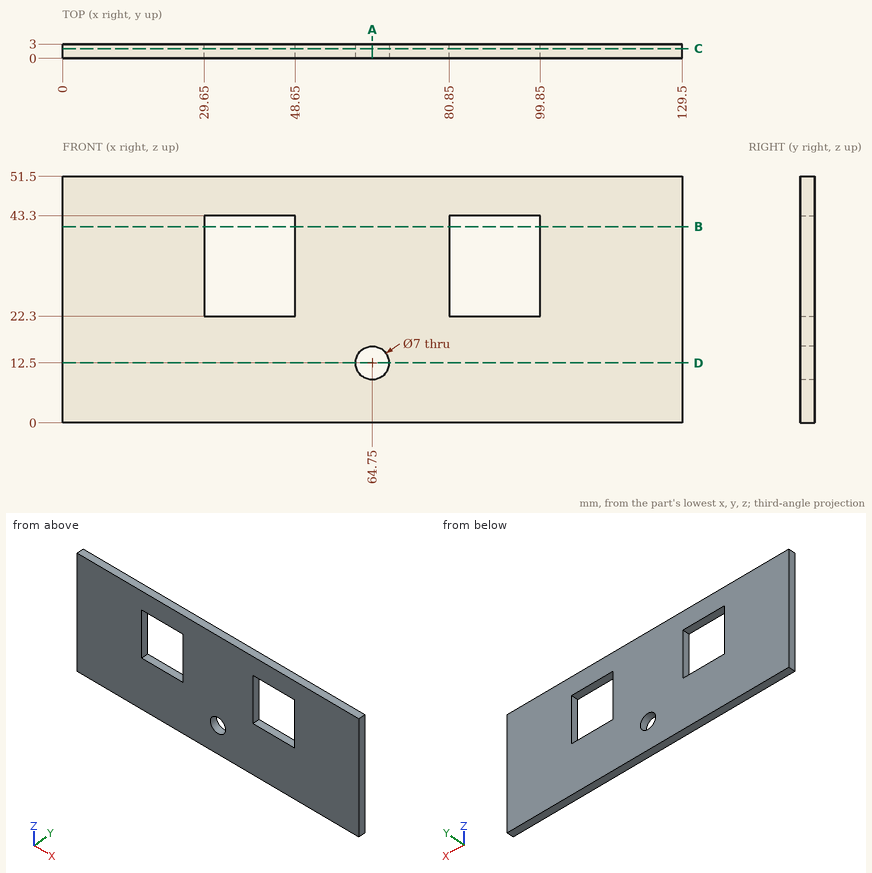
Print and shaded views of the part. All mm, measured from the part's lowest x, y and z. Coordinates: 2 decimals unless noted, no trailing zeros. Order: outer loops, then holes, each group sorted by start corner. A loop starts at its lowest first (then second) coordinate and runs counter-clockwise, first axis right, second up.
(1) Slice it at A-A, the plane x = 64.75. Write the cut outline in (y, z), and give its area (4 significant figures).
Check sheet entries:
outline: (0, 0) - (3, 0) - (3, 9) - (0, 9) - close; (0, 16) - (3, 16) - (3, 51.5) - (0, 51.5) - close
area: 133.5 mm2
(2) Slice it at D-D, the plane z = 12.5. Write the cut outline in (x, y), and give its area (4 significant figures).
Check sheet entries:
outline: (0, 0) - (61.25, 0) - (61.25, 3) - (0, 3) - close; (68.25, 0) - (129.5, 0) - (129.5, 3) - (68.25, 3) - close
area: 367.5 mm2
(3) Probe L1, parallel to X at y = 1.55, z = 41; L2, parallel to Z at x = 64.75, y = 1.45; L3, parallel to Z at x = 42, y = 1.1. List the from-to ranges inside material, lowest first.
Check sheet entries:
L1: x = 0 to 29.65, 48.65 to 80.85, 99.85 to 129.5
L2: z = 0 to 9, 16 to 51.5
L3: z = 0 to 22.3, 43.3 to 51.5
(4) Slice it at C-C, the plane y = 2.05. Write the cut outline in (x, z), and give its area (3 significant figures).
Check sheet entries:
outline: (0, 0) - (129.5, 0) - (129.5, 51.5) - (0, 51.5) - close; hole (29.65, 22.3) - (48.65, 22.3) - (48.65, 43.3) - (29.65, 43.3) - close; hole circle Ø7 at (64.75, 12.5); hole (80.85, 22.3) - (99.85, 22.3) - (99.85, 43.3) - (80.85, 43.3) - close
area: 5,830 mm2
(5) Slice it at B-B, the plane z = 41. Write the cut outline in (x, y), and give its area (4 significant figures).
Check sheet entries:
outline: (0, 0) - (29.65, 0) - (29.65, 3) - (0, 3) - close; (48.65, 0) - (80.85, 0) - (80.85, 3) - (48.65, 3) - close; (99.85, 0) - (129.5, 0) - (129.5, 3) - (99.85, 3) - close
area: 274.5 mm2
